Here's how the part is built. I have some questions about the finished solid (model axes, mm). Give positions to 0.01 mm unless a question says otherwise; leave off trailing zeros. Write each loop counter-clockwise with the first axis right and the second up, starting at its lowest first coordinate (ties: lowest second). Pieces come first, ordered by that corner, then holes. Notation, with made-up numbers: (50.25, 40.25) -> (84.25, 40.25) arc R31 cw to (84.25, 70.25) -> close; hole circle Ø7 at (55.25, -1). An arc over 180 degrees is marked (long way). Use one line per item in the form item = value.
```python
from build123d import *

# Parameters (mm, degrees)
BOSS_EXTRUDE1_DEPTH = 38.1
BOSS_EXTRUDE2_START = 10.16
SKETCH2_R           = 3.175
BOSS_EXTRUDE2_DEPTH = 10.16


with BuildPart() as part:
    # Sketch1 → Boss-Extrude1 (new body)
    with BuildSketch(Plane(origin=(0, 0, 0), x_dir=(0, 0, -1), z_dir=(1, 0, 0))):
        with BuildLine():
            Line((0.528916607, 3.130634476), (39.974911006, -3.533714773))
            ThreePointArc((39.974911006, -3.533714773), (42.576628875, -7.193265857), (38.917077791, -9.794983726))
            Line((38.917077791, -9.794983726), (-0.528916607, -3.130634476))
            ThreePointArc((-0.528916607, -3.130634476), (-3.130634476, 0.528916607), (0.528916607, 3.130634476))
        make_face()
    extrude(amount=BOSS_EXTRUDE1_DEPTH)

    # Sketch2 → Boss-Extrude2 (add)
    with BuildSketch(Plane.ZY.offset(BOSS_EXTRUDE2_START)):
        with Locations((-39.445994398, -6.664349249)):
            Circle(SKETCH2_R)
        Circle(SKETCH2_R)
    extrude(amount=-BOSS_EXTRUDE2_DEPTH)


solid = part.part
```
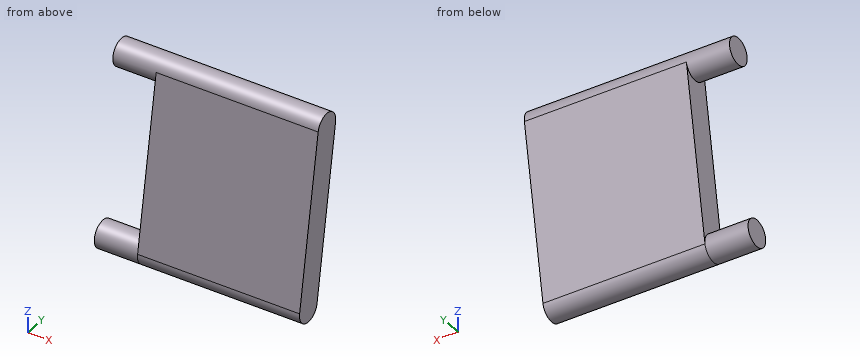
Q1. I want a section at C-C, the plane x = 13.5. Write out the boundary of the cut face in (y, z) (3 decimals), and give its area (3 significant figures).
Result set:
outline = (-9.795, -38.917) arc R3.175 ccw to (-3.534, -39.975) -> (3.131, -0.529) arc R3.175 ccw to (-3.131, 0.529) -> close
area = 286 mm2
Q2. I want a section at B-B, the plane x = -4. Write out the boundary of the cut face in (y, z) (3 decimals), and give its area (3 significant figures).
Result set:
outline = circle Ø6.35 at (-6.664, -39.446); circle Ø6.35 at (0, 0)
area = 63.3 mm2
Q3. If I drill on line 1 along X through (y, z) = (-3.5, -15.5); line 2 along Y through (x, z) = (19, -4.5); line 3 along Y through (x, z) = (23, -22.5), over which ranges is the centre line in solid material (lowest first)? Write a range as from..to.
Result set:
line_1 = 0..38.1
line_2 = -3.98..2.46
line_3 = -7.02..-0.58
Q4. Will these pins go through, and if not, where does the flat tip stop? pin 1 Ø6 at (x, z) = (2, -29) entering from -Y; pin 2 Ø6 at (x, z) = (14, -17.5) entering from +Y; pin 3 Ø3 at (x, z) = (24, -10.5) entering from -Y.
Result set:
pin_1 = -8.63
pin_2 = 0.77
pin_3 = -5.25
Q5. I want a section at A-A, the plane y = -5.75. Write out the boundary of the cut face in (x, z) (1 decimal).
Result set:
outline = (-10.2, -42.5) -> (38.1, -42.5) -> (38.1, -15) -> (0, -15) -> (0, -36.4) -> (-10.2, -36.4) -> close
Q6. I want a section at D-D, the plane z = -14. Write out the boundary of the cut face in (x, y), and give its area (3 significant figures).
Result set:
outline = (0, -5.59) -> (38.1, -5.59) -> (38.1, 0.85) -> (0, 0.85) -> close
area = 245 mm2
